Check sheet for the modelled part. Datum: model origin and axes. Units: mm. Face numbers are marked on the shaded views. Give positions to 0.01 mm unless a question says otherwise; leave off trailing zeros. Write each loop counter-clockwise with the first axis right and the second up, starting at its lowest first coordinate (ties: lowest second). Pieces come first, ordered by that corner, then holes.
from build123d import *

# Parameters (mm, degrees)
F1_DEPTH = 20
F2_R     = 11.5
F3_DEPTH = 10


with BuildPart() as f1:
    # F0 (on Top) → F1 (new body)
    with BuildSketch(Plane.XY):
        with BuildLine():
            Line((-35.837669, 47.693254), (-112.550392, -20.495833))
            Line((-112.550392, -20.495833), (-112.550392, -40.495833))
            Line((-112.550392, -40.495833), (67.449608, -40.495833))
            Line((67.449608, -40.495833), (67.449608, -20.495833))
            Line((67.449608, -20.495833), (-9.263115, 47.693254))
            ThreePointArc((-9.263115, 47.693254), (-22.550392, 52.745068), (-35.837669, 47.693254))
        make_face()
    extrude(amount=F1_DEPTH)

    # F2 (on face) → F3 (cut)
    with BuildSketch(Plane(origin=(0, 0, 0), x_dir=(1, 0, 0), z_dir=(0, 0, -1))):
        with Locations((-22.550392, -26.245068)):
            Circle(F2_R)
    extrude(amount=-F3_DEPTH, mode=Mode.SUBTRACT)


solid = f1.part
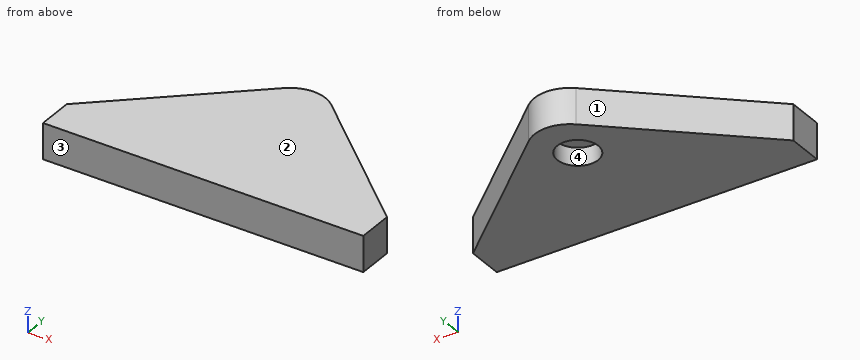
1) Sectioned sample at D-D on y = 12.5. Record the boundary of the cut face in (x, z), then the cut area to 3 significant figures.
2) Sectioned sample at B-B on z = 17.5. Record the boundary of the cut face in (x, y), then the cut area to 3 significant figures.
3) Draft check along Y on the marked faces 1, 2, 3 and 4. Enter one of: +Y half, -Y half, draft (parallel to the pull), parting line (faces both ways), or undercut.
4) Sectioned sample at A-A on z = 5. Record the boundary of the cut face in (x, y), then the cut area to 3 significant figures.
5) Sectioned sample at C-C on x = -22. Record the boundary of the cut face in (y, z), then the cut area to 3 significant figures.
6) Scan lines: L1, parallel to X at y = 17, z = 4.5; L2, parallel to Z at x = -34, y = 26.5; L3, parallel to X at y = 34.5, z = 2.5. Record each from-to range of solid material in increasing order.
7) Gauge pin test, flat ends, axial feed: pin 1 (12 mm diameter, centred on y = 1.5, z = 8.5, fed in from -X); pin 2 (3 mm diameter, centred on y = 32.5, z = 7, fed in from -X); pin 3 (10 mm diameter, centred on y = 25, z = 3, fed in from -X). Record the tip position at first contact, or that the pin passes through.
Answers below:
1. outline: (-75.43, 0) - (30.33, 0) - (30.33, 20) - (-75.43, 20) - close
1. area: 2,120 mm2
2. outline: (-112.55, -40.5) - (67.45, -40.5) - (67.45, -20.5) - (-9.26, 47.69) arc R20 ccw to (-35.84, 47.69) - (-112.55, -20.5) - close
2. area: 10,700 mm2
3. face 1: +Y half
3. face 2: draft
3. face 3: -Y half
3. face 4: undercut
4. outline: (-112.55, -40.5) - (67.45, -40.5) - (67.45, -20.5) - (-9.26, 47.69) arc R20 ccw to (-35.84, 47.69) - (-112.55, -20.5) - close; hole circle Ø23 at (-22.55, 26.25)
4. area: 10,300 mm2
5. outline: (-40.5, 0) - (14.76, 0) - (14.76, 10) - (37.73, 10) - (37.73, 0) - (52.74, 0) - (52.74, 20) - (-40.5, 20) - close
5. area: 1,630 mm2
6. L1: x = -70.37 to -29.39, -15.71 to 25.27
6. L2: z = 10 to 20
6. L3: x = -50.68 to -30.56, -14.54 to 5.58
7. pin 1: stops at x = -94.56
7. pin 2: stops at x = -54.62
7. pin 3: stops at x = -66.99
